```python
from build123d import *

# Parameters (mm, degrees)
PAD002_DEPTH        = 130
POCKET001_DEPTH     = 77
SKETCH007_R         = 2.65
HOLE002_DEPTH       = 150.001
HOLE003_D           = 5.5
HOLE003_DEPTH       = 25
HOLE003_CBORE_D     = 13
HOLE003_CBORE_DEPTH = 6.4
SKETCH011_W         = 40
SKETCH011_H         = 91
PAD003_DEPTH        = 55
POCKET002_DEPTH     = 55
POCKET002_TAPER     = 30
POCKET005_DEPTH     = 36
PAD007_DEPTH        = 54
SKETCH030_R         = 13
SKETCH030_R_2       = 10.65
POCKET010_DEPTH     = 5
POCKET012_DEPTH     = 104


with BuildPart() as part:
    # Sketch005 → Pad002 (new body)
    with BuildSketch(Plane.XY):
        Polygon((300, -70), (0, -70), (-5, -57.5), (-5, -51), (310, -51), (310, -60), align=None)
    extrude(amount=PAD002_DEPTH)

    # Sketch006 → Pocket001 (cut)
    with BuildSketch(Plane.XZ):
        Polygon((310, 60), (130, 150), (310, 150), align=None)
    extrude(amount=POCKET001_DEPTH, mode=Mode.SUBTRACT)

    # Sketch007 → Hole002 (cut, through all)
    with BuildSketch(Plane.XY.offset(150)):
        with Locations((100, -60)):
            Circle(SKETCH007_R)
        with Locations((200, -60)):
            Circle(SKETCH007_R)
        with Locations((285, -60)):
            Circle(SKETCH007_R)
        with Locations((25, -60)):
            Circle(SKETCH007_R)
    extrude(amount=-HOLE002_DEPTH, mode=Mode.SUBTRACT)

    # Hole003
    with Locations(Plane.XZ.offset(70)):
        with Locations((20, 20), (70, 20), (120, 20), (170, 20), (220, 20), (270, 20)):
            CounterBoreHole(HOLE003_D / 2, HOLE003_CBORE_D / 2, HOLE003_CBORE_DEPTH, depth=HOLE003_DEPTH)

    # Sketch011 → Pad003 (join)
    with BuildSketch(Plane.XZ):
        with Locations((15, 84.5)):
            Rectangle(SKETCH011_W, SKETCH011_H)
    extrude(amount=PAD003_DEPTH)

    # Sketch013 → Pocket002 (cut)
    with BuildSketch(Plane.XY.offset(130)):
        Polygon((-40, 30), (60, -100), (-40, -100), align=None)
    extrude(amount=-POCKET002_DEPTH, taper=POCKET002_TAPER, mode=Mode.SUBTRACT)

    # Sketch017 → Pocket005 (cut)
    with BuildSketch(Plane.YZ.offset(35)):
        Polygon((-51, 30), (0, 30), (0, 113), (-30, 113), (-51, 94), align=None)
    extrude(amount=-POCKET005_DEPTH, mode=Mode.SUBTRACT)

    # Sketch019 → Pad007 (join)
    with BuildSketch(Plane.XZ):
        Polygon((290, 70), (290, 39), (310, 39), (310, 60), align=None)
    extrude(amount=PAD007_DEPTH)

    # Sketch030 → Pocket010 (cut)
    with BuildSketch(Plane.YZ):
        with Locations((-25, 60)):
            Circle(SKETCH030_R)
        with Locations((-20, 95)):
            Circle(SKETCH030_R_2)
    extrude(amount=-POCKET010_DEPTH, mode=Mode.SUBTRACT)

    # Sketch135 → Pocket012 (cut)
    with BuildSketch(Plane.XZ):
        Polygon((-20, 140), (-20, 105), (30, 140), align=None)
    extrude(amount=POCKET012_DEPTH, mode=Mode.SUBTRACT)


with BuildPart() as part_1:
    # Body002 placement: moved
    add(part.part.moved(Location((0, 0, 10))))


solid = part_1.part
```
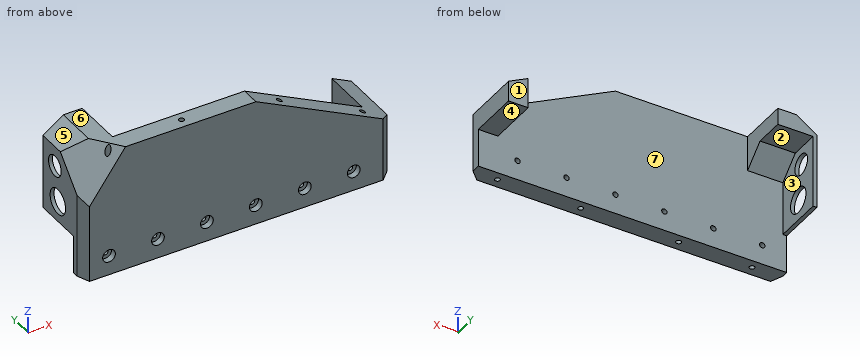
CAD build for the part. Positions are in the model's coordinates, mm. Face numbers are marked on the shaded views. A direction names the side the tool comes from. Round coordinates to 2 decimals unless told otherwise and drop trailing zeros. Write each loop counter-clockwise with the first axis right and the second up, starting at its lowest first coordinate (ties: lowest second). Pieces come first, ordered by that corner, then holes. Notation, with made-up numbers: (75, -1) - (81, -1) arc R10 ccw to (81, 9) - close; hole circle Ø1 at (47, 29.5). An arc over 180 degrees is marked (long way). Return JSON: item names as keys, results as strings. Group by question number.
Item 1: Band-saw the part on C-C on x = 251.5. List the corners of the cut face in (y, z), plus the area to 3 significant figures.
Item 2: Band-saw the part on B-B on x = 133. List the corners of the cut face in (y, z), plus the area to 3 significant figures.
Item 3: Mould opens along X. For the marked faces 5, 6 and 7 say: +X half, -X half, draft (parallel to the pull), parting line (faces both ways), or undercut.
Item 4: 3-axis set-ups, long thin cutter, end or side, ignore diameter. For the marked faces 1, 2, 3 and 4: which of +Z, -Z, +X, -X, +Y, -Y reach the whole face in a straight line?
Item 5: Flat gauge pins, fed straight in: pin 1 Ø3 at (x, z) = (264, 82) entering from +Y; pin 2 Ø4 at (x, z) = (69.5, 29) entering from -Y; pin 3 Ø7 at (x, y) = (285, -60) entering from +Z; pin 4 Ø10.5 at (x, z) = (21.5, 27.5) entering from -Y. Where does each tip first touch, or does it go through?
Item 6: Probe probe 1 along Y at (x, z) = (285, 43); probe 2 along X at (y, z) = (-58, 113.5); probe 3 along X at (y, z) = (-31.5, 54). List the from-to ranges inside material, lowest first.
Item 7: Band-saw the part on A-A on y = -25. List the corners of the cut face in (x, z).
Resolved:
{
 "1": {"outline": "(-70, 10) - (-51, 10) - (-51, 99.25) - (-70, 99.25) - close", "area": "1,700 mm²"},
 "2": {"outline": "(-70, 10) - (-51, 10) - (-51, 140) - (-70, 140) - close", "area": "2,470 mm²"},
 "3": {"face 5": "-X half", "face 6": "draft", "face 7": "undercut"},
 "4": {"face 1": "+Z, -Z, +X, -X, +Y", "face 2": "-Z, +X, +Y", "face 3": "-Z, +Y", "face 4": "-Z, +X, -X, +Y"},
 "5": {"pin 1": "stops at y = -51", "pin 2": "stops at y = -63.6", "pin 3": "stops at z = 84.25", "pin 4": "stops at y = -70"},
 "6": {"probe 1": "y = -70 to -62.65, -57.35 to -51", "probe 2": "x = 8.39 to 23.26, 26.74 to 98.26, 101.74 to 198.26, 201.74 to 223", "probe 3": "x = -5 to -1, 290 to 310"},
 "7": {"outline": "(-5, 49) - (-1, 49) - (-1, 57) - (-5, 57) - close; (-5, 83) - (-1, 83) - (-1, 95.6) - (-5, 95.6) - close; (-5, 114.4) - (-1, 114.4) - (-1, 123) - (35, 123) - (35, 140) - (15.71, 140) - (-5, 125.5) - close; (290, 49) - (310, 49) - (310, 70) - (290, 80) - close"}
}
